from build123d import *

# Parameters (mm, degrees)
SKETCH1_R           = 2
BOSS_EXTRUDE1_DEPTH = 40
SKETCH2_R           = 2.633085966
BOSS_EXTRUDE2_DEPTH = 1
FILLET1_R           = 1
BOSS_EXTRUDE3_START = 1
SKETCH3_R           = 2.633085966
BOSS_EXTRUDE3_DEPTH = 1
FILLET2_R           = 1


with BuildPart() as part:
    # Sketch1 → Boss-Extrude1 (new body)
    with BuildSketch(Plane(origin=(0, 0, 0), x_dir=(1, 0, 0), z_dir=(0, 1, 0))):
        with Locations(Location((0, 0, 0), (0, 0, 90))):
            Circle(SKETCH1_R)
    extrude(amount=BOSS_EXTRUDE1_DEPTH)

    # Sketch2 → Boss-Extrude2 (add)
    with BuildSketch(Plane(origin=(0, 40, 0), x_dir=(1, 0, 0), z_dir=(0, 1, 0))):
        Circle(SKETCH2_R)
    extrude(amount=BOSS_EXTRUDE2_DEPTH)

    # Fillet1
    fillet1_edges = [part.edges().sort_by_distance(p)[0] for p in [
        (-2.633085966, 41, 0),
    ]]
    fillet(fillet1_edges, radius=FILLET1_R - 0.0001)  # a hair under: the kernel refuses the full size

    # Sketch3 → Boss-Extrude3 (add)
    with BuildSketch(Plane.XZ.offset(BOSS_EXTRUDE3_START)):
        Circle(SKETCH3_R)
    extrude(amount=-BOSS_EXTRUDE3_DEPTH)

    # Fillet2
    fillet2_edges = [part.edges().sort_by_distance(p)[0] for p in [
        (-2.633085966, -1, 0),
    ]]
    fillet(fillet2_edges, radius=FILLET2_R - 0.0001)  # a hair under: the kernel refuses the full size


solid = part.part
For this review, take the finished solid that the model builds, in its own axes (mm). Round coordinates to 2 decimals unless told otherwise and drop trailing zeros. Loops run counter-clockwise (first coordinate to the right, second up) from the corner with the lowest first, then second, coordinate; pieces in that order, holes last. Notation, with made-up numbers: (68, 30) - (88, 30) arc R21 ccw to (88, 63) - close; hole circle Ø11 at (-35, 16). An arc over 180 degrees is marked (long way). Put each result on its own line as item: value. Start each with the question number.
1. Mouldability with a two-part tool opening along Y and no side actions: class faces 1 (the flat face through (2, 40, -1)), 2 (the flat face through (0, -1, 0)), 3 (the flat face through (0, 41, 0)) as +Y half, -Y half, draft (parallel to the pull), parting line (faces both ways), or undercut.
2. Consider section C-C on y = 33. State the section outline as (x, z) points, plus the area to 3 significant figures.
3. Insertion check: P1, Ø2, axis at x = 1.5, y = 11, coming from the -Z side; P2, Ø1.5, axis at y = 32, z = 2, coming from the -X side; P3, Ø1, axis at x = -1.5, y = 6.5, coming from the -Z side. Each pin has a flat end and moves straight along its axis. Give the tip position at first contact, or say it passes through.
4. For probe 1 along Y at (x, z) = (-1.05, 1.9); probe 2 along Y at (x, z) = (-0.1, 1.75); probe 3 along Y at (x, z) = (0.35, -2.4), list the stretches that pass through material, from the lowest coordinate up. Write a range as [from, to].
Result sheet:
1. face 1: undercut
1. face 2: -Y half
1. face 3: +Y half
2. outline: circle Ø4 at (0, 0)
2. area: 12.6 mm^2
3. P1: z = -1.94
3. P2: x = -1.56
3. P3: z = -1.73
4. probe 1: [-0.84, 0], [40, 40.84]
4. probe 2: [-0.99, 40.99]
4. probe 3: [-0.61, 0], [40, 40.61]
